Autodesk Inventor part; units mm, degrees
ref_plane "Work Plane1" through (0, 0, 0) normal (0, 0, 1) x (1, 0, 0)
ref_plane "YZ Plane" through (0, 0, 0) normal (1, 0, 0) x (0, 1, 0)
ref_plane "XZ Plane" through (0, 0, 0) normal (0, 1, 0) x (-1, 0, 0)
ref_plane "Work Plane1" through (0, 0, 0) normal (0, 0, 1) x (1, 0, 0)
sketch "Sketch1" plane through (0, 0, 0) normal (0, 0, 1) x (1, 0, 0)
  arc A0 (63.0305, 195.3497) -> (48.9551, 209.4251) centre (68.2595, 214.6541) ccw
  circle A1 centre (68.2595, 214.6541) radius 4.25
  circle A2 centre (68.2595, 214.6541) radius 20
  point P0 (0, 0)
  point P1 (28.2595, 174.6541)
  dimension "d1" = 40
  dimension "d2" = 8.5
extrude "Extrusion1" add sketch "Sketch1" along normal blind 6
chamfer "Chamfer1" distance 5 angle 45 1 edges at (82.4016, 228.7962, 6)
properties part number "plastic_wheel_washer"
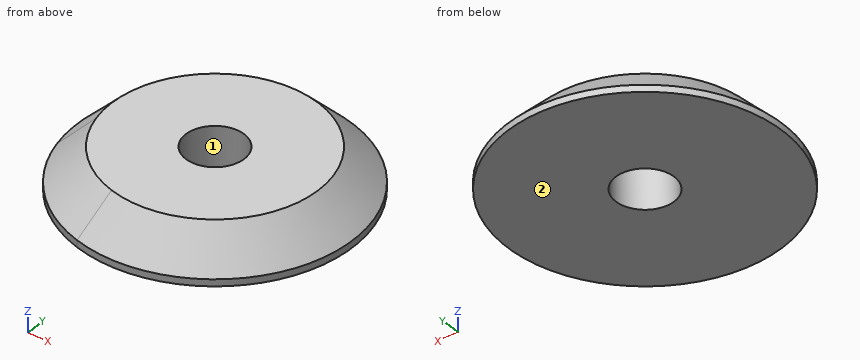
For this review, take the finished solid that the model builds, in its own axes (mm). Face numbers are marked on the shaded views. Round coordinates to 2 decimals unless told otherwise and drop trailing zeros. Order: outer loops, then holes, each group sorted by start corner. A loop starts at its lowest first (then second) coordinate and runs counter-clockwise, first axis right, second up. Notation, with made-up numbers: M 38.5,-33 L 75.5,-33 A21 ccw 75.5,-29 Z; hole C -7,85 d3. An arc over 180 degrees is marked long. Write each question's results on one line, items separated by ' | '. Start each with the question number.
1. To check wall thickness, follow L1, parallel to X at y = 218.5, z = 2.45; L2, parallel to Y at x = 72, z = 4.2; L3, parallel to Y at x = 71, z = 3.6. State the ranges of each line that lie inside material, in increasing order. Write a range as [from, to].
2. Add section B-B (z = 1.9). State the section outline as (x, y) points.
3. Clearance check with flat-ended pins moving along their axes: pin 1 Ø12 at (x, y) = (84, 229) entering from +Z; pin 2 Ø2 at (x, z) = (72, 2) entering from -Y; pin 3 Ø1 at (x, z) = (64, 2) entering from -Y; pin 4 Ø2 at (x, y) = (70, 221) entering from -Z. State where each tip first meets the part, or that it passes through.
4. Add section A-A (z = 4.8). State the section outline as (x, y) points, then the cut area to 3 significant figures.
5. Draft analysis for pull direction Y (two halves, no side actions). For the marked faces 1 and 2, state which applies: pulls with the +Y half, pulls with the -Y half, needs draft (parallel to the pull), parting line crosses it, or undercut.
Output values:
1) L1: [50.11, 66.45], [70.07, 86.41] | L2: [198.28, 212.64], [216.67, 231.03] | L3: [197.47, 211.41], [217.9, 231.84]
2) outline: M 49.82,209.66 A19.1 ccw 63.27,196.22 A19.1 ccw long Z; hole C 68.26,214.65 d8.5
3) pin 1: z = 5.7 | pin 2: y = 194.99 | pin 3: y = 195.61 | pin 4: z = 0
4) outline: M 52.62,210.42 A16.2 ccw 64.02,199.02 A16.2 ccw long Z; hole C 68.26,214.65 d8.5 | area: 768 mm^2
5) face 1: undercut | face 2: needs draft
